from build123d import *

# Parameters (mm, degrees)
SKETCH1_R           = 5.7785
BOSS_EXTRUDE1_DEPTH = 25.4
SKETCH2_R           = 2.921
CUT_EXTRUDE1_DEPTH  = 27.513623
SKETCH3_W           = 5.969
SKETCH3_H           = 4.005387026
CUT_EXTRUDE2_DEPTH  = 26.4000001
FILLET1_R           = 1.27
FILLET2_R           = 1.27


with BuildPart() as part:
    # Sketch1 → Boss-Extrude1 (new body)
    with BuildSketch(Plane(origin=(0, 0, 0), x_dir=(0, 0, -1), z_dir=(1, 0, 0))):
        with BuildLine():
            Line((-8.9535, 19.05), (-8.9535, 0))
            ThreePointArc((-8.9535, 0), (0, -8.9535), (8.9535, 0))
            Line((8.9535, 0), (8.9535, 19.05))
            Line((8.9535, 19.05), (-8.9535, 19.05))
        make_face()
        Circle(SKETCH1_R, mode=Mode.SUBTRACT)
    extrude(amount=BOSS_EXTRUDE1_DEPTH)

    # Sketch2 → Cut-Extrude1 (cut)
    with BuildSketch(Plane(origin=(0, 19.05, 0), x_dir=(1, 0, 0), z_dir=(0, 1, 0))):
        with Locations((6.35, 0)):
            Circle(SKETCH2_R)
        with Locations((19.05, 0)):
            Circle(SKETCH2_R)
    extrude(amount=-CUT_EXTRUDE1_DEPTH, mode=Mode.SUBTRACT)

    # Sketch3 → Cut-Extrude2 (cut, through all)
    with BuildSketch(Plane.ZY):
        with Locations((0, -6.950806487)):
            Rectangle(SKETCH3_W, SKETCH3_H)
    extrude(amount=-CUT_EXTRUDE2_DEPTH, mode=Mode.SUBTRACT)

    # Fillet1
    fillet1_edges = [part.edges().sort_by_distance(p)[0] for p in [
        (0, 5.031748975, 2.84122588),
        (0, -6.694776864, 2.9845),
        (25.4, 5.031748975, 2.84122588),
        (0, -6.694776864, -2.9845),
        (25.4, -6.694776864, -2.9845),
        (25.4, -6.694776864, 2.9845),
    ]]
    fillet(fillet1_edges, radius=FILLET1_R)

    # Fillet2
    fillet2_edges = [part.edges().sort_by_distance(p)[0] for p in [
        (12.7, 19.05, 8.9535),
        (12.7, 19.05, -8.9535),
        (25.4, 19.05, 0),
        (0, 19.05, 0),
    ]]
    fillet(fillet2_edges, radius=FILLET2_R)


solid = part.part
Verification items for the finished model (mm, model axes). A direction names the side the tool comes from. Give positions to 0.01 mm unless a question says otherwise; leave off trailing zeros. Order: outer loops, then holes, each group sorted by start corner. A loop starts at its lowest first (then second) coordinate and runs counter-clockwise, first axis right, second up. Notation, with made-up numbers: M 67.25,-10 L 88.25,-10 A12 ccw 88.25,-5 Z; hole C 26.5,85.5 d8. An arc over 180 degrees is marked long. Answer as a JSON object with one key per item and string values. Group by question number.
1) Cross-section at D-D (y = 14.75). Enter the section's corners in (x, z), then the cut area to 3 significant figures.
2) Cross-section at C-C (x = 10.25). Enter the section's corners in (y, z), then the cut area to 3 significant figures.
3) Cross-section at B-B (x = 19.05). Enter the section's corners in (y, z).
4) Cross-section at A-A (z = 0). Enter the section's corners in (x, y).
5) Access from +Z, -Z, +X, -X, +Y, -Y to the whole of each face (thin tool, end or side, straight path). Record for faces 1 (the face through (0.36, -6.67, 3.37)), 2 (the face through (12.52, -5.11, 7.35)), 3 (the face through (12.522, -5.232, -7.266)), 4 (the face through (25.04, -6.72, 3.37)), 5 (the face through (13, -7, 2.984)).
6) Scan lines: line 1 along X through (y, z) = (12.5, 0); line 2 along Z through (x, y) = (22.75, -0.25); line 3 along Z through (x, y) = (19.05, 9). Record each from-to range of solid material in increasing order. Write a range as [from, to].
7) Depth check by flat-ended pin: pin 1 Ø2 at (x, z) = (12, 0.5) entering from -Y; pin 2 Ø4 at (x, z) = (3.5, -4.5) entering from -Y; pin 3 Ø4.5 at (x, z) = (6.35, 0) entering from -Y; pin 4 Ø3 at (x, y) = (11.5, -6.5) entering from -Z. Enter the tip coordinate at first touch or a pass-through.
Result sheet:
{
 "1": {"outline": "M 0,-8.95 L 25.4,-8.95 L 25.4,8.95 L 0,8.95 Z; hole C 6.35,0 d5.84; hole C 19.05,0 d5.84", "area": "401 mm2"},
 "2": {"outline": "M -8.44,-2.98 A8.95 ccw 0,-8.95 L 17.78,-8.95 A1.27 ccw 19.05,-7.68 L 19.05,7.68 A1.27 ccw 17.78,8.95 L 0,8.95 A8.95 ccw -8.44,2.98 L -4.95,2.98 A5.78 cw long -4.95,-2.98 Z", "area": "342 mm2"},
 "3": {"outline": "M -8.44,-2.98 A8.95 ccw 0,-8.95 L 17.78,-8.95 A1.27 ccw 19.05,-7.68 L 19.05,-2.92 L 4.99,-2.92 A5.78 cw -4.95,-2.98 Z; M -8.44,2.98 L -4.95,2.98 A5.78 cw 4.99,2.92 L 19.05,2.92 L 19.05,7.68 A1.27 ccw 17.78,8.95 L 0,8.95 A8.95 ccw Z"},
 "4": {"outline": "M 0,7.05 A1.27 ccw 1.27,5.78 L 3.43,5.78 L 3.43,19.05 L 1.27,19.05 A1.27 ccw 0,17.78 Z; M 9.27,5.78 L 16.13,5.78 L 16.13,19.05 L 9.27,19.05 Z; M 21.97,5.78 L 24.13,5.78 A1.27 ccw 25.4,7.05 L 25.4,17.78 A1.27 ccw 24.13,19.05 L 21.97,19.05 Z"},
 "5": {"face 1": "-X, -Y", "face 2": "+Z, +X, -X, -Y", "face 3": "-Z, +X, -X, -Y", "face 4": "+X, -Y", "face 5": "+X, -X, -Y"},
 "6": {"line 1": "x = [0, 3.43], [9.27, 16.13], [21.97, 25.4]", "line 2": "z = [-8.95, -5.77], [5.77, 8.95]", "line 3": "z = [-8.95, -2.92], [2.92, 8.95]"},
 "7": {"pin 1": "stops at y = 5.58", "pin 2": "stops at y = -8.44", "pin 3": "passes through", "pin 4": "stops at z = -7.43"}
}
